```python
from build123d import *

# Parameters (mm, degrees)
PAD_DEPTH         = 150
FILLET_R          = 4
FILLET001_R       = 1.9
FILLET002_R       = 10
FILLET003_R       = 8
FILLET004_R       = 8
FILLET005_R       = 6
FILLET006_R       = 8
FILLET007_R       = 6
FILLET008_R       = 4
FILLET009_R       = 7
FILLET010_R       = 5
FILLET011_R       = 6
FILLET012_R       = 5
SKETCH003_R       = 16
SKETCH003_R_2     = 13
PAD001_DEPTH      = 150
SKETCH004_R       = 2.5
HOLE_DEPTH        = 77.001
CHAMFER_SIZE      = 1
POCKET_DEPTH      = 78.001
POCKET_DEPTH_BACK = 1.634975


with BuildPart() as part:
    # Sketch001 → Pad (new body)
    with BuildSketch(Plane.YZ):
        Polygon((77, -10), (35.375644, -10), (-4.098076, 58.37049), (4.562178, 63.37049), (26.081416, 26.098076), (43.401924, 36.098076), (0, 111.272413), (8.660254, 116.272413), (30.411543, 78.598076), (43.401924, 86.098076), (0, 161.272413), (8.660254, 166.272413), (30.411543, 128.598076), (43.401924, 136.098076), (0, 211.272413), (8.660254, 216.272413), (30.411543, 178.598076), (43.401924, 186.098076), (0, 261.272413), (8.660254, 266.272413), (61.009619, 175.600654), (74, 183.100654), (52.696152, 220), (77, 220), align=None)
        Polygon((37.107695, -7), (27.292741, 10), (74, 10), (74, -7), align=None, mode=Mode.SUBTRACT)
        Polygon((0, 57.272413), (3.464102, 59.272413), (24.98334, 22), (47.5, 35), (4.098076, 110.174337), (7.562178, 112.174337), (29.313467, 74.5), (47.5, 85), (4.098076, 160.174337), (7.562178, 162.174337), (29.313467, 124.5), (47.5, 135), (4.098076, 210.174337), (7.562178, 212.174337), (29.313467, 174.5), (47.5, 185), (4.098076, 260.174337), (7.562178, 262.174337), (59.911543, 171.502577), (74, 179.636552), (74, 13), (25.56069, 13), align=None, mode=Mode.SUBTRACT)
        Polygon((74, 189.100654), (57.892305, 217), (74, 217), align=None, mode=Mode.SUBTRACT)
    extrude(amount=PAD_DEPTH)

    # Fillet
    fillet_edges = [part.edges().sort_by_distance(p)[0] for p in [
        (75, -4.098076, 58.37049),
        (75, 4.562178, 63.37049),
        (75, 0, 111.272413),
        (75, 8.660254, 116.272413),
        (75, 0, 161.272413),
        (75, 8.660254, 166.272413),
        (75, 0, 211.272413),
        (75, 8.660254, 216.272413),
        (75, 0, 261.272413),
        (75, 8.660254, 266.272413),
    ]]
    fillet(fillet_edges, radius=FILLET_R)

    # Fillet001
    fillet001_edges = [part.edges().sort_by_distance(p)[0] for p in [
        (75, 3.464102, 59.272413),
        (75, 0, 57.272413),
        (75, 7.562178, 112.174337),
        (75, 4.098076, 110.174337),
        (75, 4.098076, 160.174337),
        (75, 7.562178, 162.174337),
        (75, 7.562178, 212.174337),
        (75, 4.098076, 210.174337),
        (75, 7.562178, 262.174337),
        (75, 4.098076, 260.174337),
    ]]
    fillet(fillet001_edges, radius=FILLET001_R)

    # Fillet002
    fillet002_edges = [part.edges().sort_by_distance(p)[0] for p in [
        (75, 47.5, 35),
        (75, 24.98334, 22),
    ]]
    fillet(fillet002_edges, radius=FILLET002_R)

    # Fillet003
    fillet003_edges = [part.edges().sort_by_distance(p)[0] for p in [
        (75, 43.401924, 36.098076),
        (75, 26.081416, 26.098076),
    ]]
    fillet(fillet003_edges, radius=FILLET003_R)

    # Fillet004
    fillet004_edges = [part.edges().sort_by_distance(p)[0] for p in [
        (75, 47.5, 85),
        (75, 29.313467, 74.5),
        (75, 29.313467, 124.5),
        (75, 47.5, 135),
        (75, 29.313467, 174.5),
        (75, 47.5, 185),
    ]]
    fillet(fillet004_edges, radius=FILLET004_R)

    # Fillet005
    fillet005_edges = [part.edges().sort_by_distance(p)[0] for p in [
        (75, 30.411543, 128.598076),
        (75, 30.411543, 78.598076),
        (75, 43.401924, 86.098076),
        (75, 43.401924, 136.098076),
        (75, 30.411543, 178.598076),
        (75, 43.401924, 186.098076),
    ]]
    fillet(fillet005_edges, radius=FILLET005_R)

    # Fillet006
    fillet006_edges = [part.edges().sort_by_distance(p)[0] for p in [
        (75, 59.911543, 171.502577),
    ]]
    fillet(fillet006_edges, radius=FILLET006_R)

    # Fillet007
    fillet007_edges = [part.edges().sort_by_distance(p)[0] for p in [
        (75, 61.009619, 175.600654),
        (75, 74, 183.100654),
    ]]
    fillet(fillet007_edges, radius=FILLET007_R)

    # Fillet008
    fillet008_edges = [part.edges().sort_by_distance(p)[0] for p in [
        (75, 57.892305, 217),
        (75, 74, 217),
    ]]
    fillet(fillet008_edges, radius=FILLET008_R)

    # Fillet009
    fillet009_edges = [part.edges().sort_by_distance(p)[0] for p in [
        (75, 52.696152, 220),
        (75, 77, 220),
    ]]
    fillet(fillet009_edges, radius=FILLET009_R)

    # Fillet010
    fillet010_edges = [part.edges().sort_by_distance(p)[0] for p in [
        (75, 74, 13),
        (75, 25.56069, 13),
        (75, 74, 10),
        (75, 27.292741, 10),
        (75, 37.107695, -7),
        (75, 74, -7),
    ]]
    fillet(fillet010_edges, radius=FILLET010_R)

    # Fillet011
    fillet011_edges = [part.edges().sort_by_distance(p)[0] for p in [
        (75, 77, -10),
    ]]
    fillet(fillet011_edges, radius=FILLET011_R)

    # Fillet012
    fillet012_edges = [part.edges().sort_by_distance(p)[0] for p in [
        (75, 35.375644, -10),
    ]]
    fillet(fillet012_edges, radius=FILLET012_R)

    # Sketch003 → Pad001 (join)
    with BuildSketch(Plane.YZ):
        with Locations((59, 82)):
            Circle(SKETCH003_R)
        with Locations((59, 82)):
            Circle(SKETCH003_R_2, mode=Mode.SUBTRACT)
    extrude(amount=PAD001_DEPTH)

    # Sketch004 → Hole (cut, through all)
    with BuildSketch(Plane.XZ):
        with Locations((37.5, 173.754105)):
            Circle(SKETCH004_R)
        with Locations((112.5, 173.754105)):
            Circle(SKETCH004_R)
    extrude(amount=-HOLE_DEPTH, mode=Mode.SUBTRACT)

    # Chamfer
    chamfer_edges = [part.edges().sort_by_distance(p)[0] for p in [
        (110, 74, 173.754105),
        (35, 74, 173.754105),
    ]]
    chamfer(chamfer_edges, length=CHAMFER_SIZE)

    # Sketch002 → Pocket (cut, two sides)
    with BuildSketch(Plane.XZ.offset(1)) as pocket_sk:
        Polygon((0, -19.218618), (0, 278.271382), (50, -19.218618), align=None)
    extrude(amount=-POCKET_DEPTH, mode=Mode.SUBTRACT)
    extrude(pocket_sk.sketch, amount=POCKET_DEPTH_BACK, mode=Mode.SUBTRACT)


solid = part.part
```
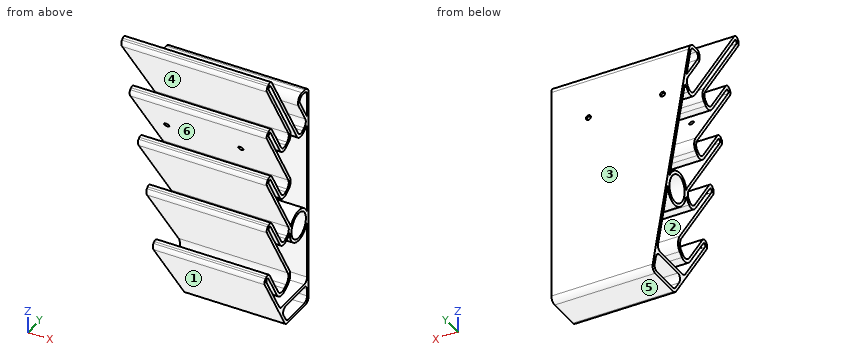
Check sheet for the modelled part. Datum: model origin and axes. Units: mm. Face numbers are marked on the shaded views. A direction names the side the tool comes from. Give positions to 0.01 mm unless a question says otherwise; leave off trailing zeros. Loops run counter-clockwise (first coordinate to the right, second up) from the corner with the lowest first, then second, coordinate; pieces in that order, holes last. Notation, with made-up numbers: M 47.5,-32.5 L 88.5,-32.5 A11 ccw 88.5,-28.5 Z; hole C 65,-34.75 d1. An arc over 180 degrees is marked long. Answer in a Markdown table with one row per item.
1) Cross-section at B-B (z = 148). Enter the section's corners in (x, y), plus the area to 3 significant figures.
Solutions:
| item | result |
|---|---|
| outline | M 21.9,7.66 L 150,7.66 L 150,11.13 L 21.9,11.13 Z; M 21.9,15.75 L 150,15.75 L 150,19.21 L 21.9,19.21 Z; M 21.9,36.53 L 150,36.53 L 150,39.99 L 21.9,39.99 Z; M 21.9,74 L 150,74 L 150,77 L 21.9,77 Z |
| area | 1,720 mm^2 |
2) Depth check by flat-ended pin: pin 1 (8 mm diameter, centred on x = 51, y = 27.5, fed in from -Z); pin 2 (8 mm diameter, centred on x = 35, z = 119, fed in from -Y); pin 3 (1 mm diameter, centred on x = 96.5, y = 16.5, fed in from -Z). Enter the tip coordinate at first touch or a pass-through.
Solutions:
| item | result |
|---|---|
| pin 1 | stops at z = -3.29 |
| pin 2 | stops at y = 22.1 |
| pin 3 | stops at z = 21.83 |
3) Thickness scan on line 1 (Y direction, x = 85, z = 145); line 2 (Y direction, x = 51, z = 155); line 3 (Z direction, x = 70, y = 49). Record the ranges inside material, lowest first.
Solutions:
| item | result |
|---|---|
| line 1 | y = 9.39 to 12.86, 17.48 to 20.94, 38.26 to 41.73, 74 to 77 |
| line 2 | y = 3.62 to 7.09, 11.7 to 15.17, 32.49 to 35.95, 74 to 77 |
| line 3 | z = -10 to -7, 10 to 13, 69.51 to 73.69, 90.31 to 94.49, 190.4 to 196.4 |
4) Cross-section at A-A (z = 245.5). Enter the section's corners in (x, y).
Solutions:
| item | result |
|---|---|
| outline | M 5.51,9.11 L 150,9.11 L 150,12.57 L 5.51,12.57 Z; M 5.51,17.19 L 150,17.19 L 150,20.65 L 5.51,20.65 Z |
5) Mould release check, pull along Z, two halves, no side actions. Record for the marked faces 1, 2, 3 and 4: released by +Z, released by -Z, zero draft, split by the parting line, or undercut.
Solutions:
| item | result |
|---|---|
| face 1 | released by -Z |
| face 2 | undercut |
| face 3 | zero draft |
| face 4 | undercut |
6) Cross-section at C-C (x = 120.5). Count the separate pieces of the cut face and the enclosed holes in it, plus the area to 3 significant figures.
Solutions:
| item | result |
|---|---|
| separate pieces | 1 |
| enclosed holes | 5 |
| area | 3,790 mm^2 |
7) Tool access check on the marked faces 5 and 6. Record the directions out of +Z, -Z, +X, -X, +Y, -Y that give a thin tool (end or side, any length) a straight path to the whole face; none if there is none.
Solutions:
| item | result |
|---|---|
| face 5 | -Z, +X, -X, +Y, -Y |
| face 6 | +X, -X |
